Check sheet for the modelled part. Datum: model origin and axes. Units: mm. Round coordinates to 2 decimals unless told otherwise and drop trailing zeros. Write each loop counter-clockwise with the first axis right and the second up, starting at its lowest first coordinate (ties: lowest second). Pieces come first, ordered by that corner, then holes.
Item 1: Release check for a two-part mould opening along Z. For faces 1 (the flat face through (-2, 10, 6)), 2 (the cylindrical face through (2.4, 5.1, 4.5)), 3 (the flat face through (4.44, 4.93, 7.83)), 4 (the conical face through (8.08, 9.8, -4.69)) record: pulls with the +Z half, pulls with the -Z half, needs draft (parallel to the pull), parting line crosses it, or undercut.
Item 2: Section check A-A, the plane y = 16. Record the cut outline in (x, z), plus the area to 3 significant figures.
Item 3: Depth check by flat-ended pin: pin 1 (4 mm diameter, centred on x = 6, y = 9, fed in from +Z); pin 2 (10 mm diameter, centred on x = -6.5, y = 7.5, fed in from +Z); pin 3 (1.5 mm diameter, centred on y = 12.5, z = 8, fed in from +X). Enter the tip coordinate at first touch or a pass-through.
Item 4: Material ranges on line 1 along X through (y, z) = (3.5, 0); line 2 along Y through (x, z) = (7, 1.25); line 3 along X through (y, z) = (9.25, 0.75), recorded low to high.
from build123d import *

# Parameters (mm, degrees)
EXTRUDE_1_DEPTH     = 10
HOLE_WIZARD_M12_1_D = 10.2
CHAMFER_2_SIZE      = 1


with BuildPart() as part:
    # 草图1 → 凸台-拉伸1 (new body)
    with BuildSketch(Plane(origin=(0, 0, 0), x_dir=(1, 0, 0), z_dir=(0, 1, 0))):
        Polygon((9, -5.196152423), (9, 5.196152423), (0, 10.392304845), (-9, 5.196152423), (-9, -5.196152423), (0, -10.392304845), align=None)
    extrude(amount=EXTRUDE_1_DEPTH)

    # 草图3 → 切除-旋转1 (revolve, cut)
    with BuildSketch(Plane(origin=(0, 0, 0), x_dir=(0, 0, -1), z_dir=(1, 0, 0))):
        Polygon((9, 10), (10.392304845, 9.196152423), (10.392304845, 10), align=None)
    cut_revolve_1 = revolve(axis=Axis((0, 12.408393564, 0), (0, -1, 0)), mode=Mode.SUBTRACT)

    # 镜向1: 切除-旋转1 across plane
    add(cut_revolve_1.mirror(Plane.ZX.offset(5)), mode=Mode.SUBTRACT)

    # M12 螺纹孔1 (through all)
    with Locations(Plane(origin=(0, 0, 0), x_dir=(-1, 0, 0), z_dir=(0, -1, 0))):
        with Locations((0, 0)):
            Hole(HOLE_WIZARD_M12_1_D / 2)

    # 倒角2
    chamfer_2_edges = [part.edges().sort_by_distance(p)[0] for p in [
        (-5.1, 0, 0),
        (-5.1, 10, 0),
    ]]
    chamfer(chamfer_2_edges, length=CHAMFER_2_SIZE)

    # 草图9 → 旋转-薄壁1 (revolve)
    with BuildSketch(Plane(origin=(0, 0, 0), x_dir=(0, 0, -1), z_dir=(1, 0, 0)), mode=Mode.PRIVATE) as revolve_1_sk:
        with BuildLine():
            ThreePointArc((0, 19), (6.363961031, 16.363961031), (9, 10))
            Line((9, 10), (8, 10))
            ThreePointArc((8, 10), (5.656854249, 15.656854249), (0, 18))
            Line((0, 18), (0, 19))
        make_face()
    revolve(revolve_1_sk.sketch.rotate(Axis((0, 21.479292142, 0), (0, -1, 0)), 180), axis=Axis((0, 21.479292142, 0), (0, -1, 0)))


solid = part.part
Values found:
1. face 1: undercut
1. face 2: undercut
1. face 3: pulls with the +Z half
1. face 4: pulls with the -Z half
2. outline: circle Ø13.42 at (0, 0); hole circle Ø10.58 at (0, 0)
2. area: 53.4 mm2
3. pin 1: stops at z = 8.08
3. pin 2: stops at z = 9.53
3. pin 3: stops at x = 4.77
4. line 1: x = -9 to -5.1, 5.1 to 9
4. line 2: y = 0 to 10, 13.67 to 15.52
4. line 3: x = -9 to -5.3, 5.3 to 9
